from build123d import *

# Parameters (mm, degrees)
F0_R     = 20
F0_R_2   = 15
F1_DEPTH = 34
F2_R     = 22
F2_R_2   = 12
F3_DEPTH = 10.414


# Not quite as in the source:
# - a pattern or mirror of a feature is missing from the dataset's text; its kind, count and spacing are read off the source's solid


with BuildPart() as f1:
    # F0 (on Right) → F1 (new body, symmetric)
    with BuildSketch(Plane.YZ):
        Circle(F0_R)
        Circle(F0_R_2, mode=Mode.SUBTRACT)
    extrude(amount=F1_DEPTH, both=True)

    # F2 (on face) → F3 (join)
    with BuildSketch(Plane.YZ.offset(34)):
        Circle(F2_R)
        Circle(F2_R_2, mode=Mode.SUBTRACT)
    f3 = extrude(amount=F3_DEPTH)

    # F3_copies: F3 across plane
    add(f3.mirror(Plane(origin=(0, 0, 0), x_dir=(0, 0, -1), z_dir=(-1, 0, 0))))


solid = f1.part
Design review of the part built by this model. Coordinates are the model's own, in mm. A direction names the side the tool comes from. Give positions to 0.01 mm unless a question says otherwise; leave off trailing zeros. Write each loop counter-clockwise with the first axis right and the second up, starting at its lowest first coordinate (ties: lowest second). Pieces come first, ordered by that corner, then holes. Notation, with made-up numbers: M 53.25,64 L 111.25,64 A12 cw 111.25,70 Z; hole C -7.5,-5 d11. An arc over 180 degrees is marked long. Return JSON: item names as keys, results as strings. Group by question number.
Item 1: Clearance check with flat-ended pins moving along their axes: pin 1 Ø5 at (x, z) = (-33, -10.5) entering from +Y; pin 2 Ø6 at (x, z) = (30, -16.5) entering from -Y; pin 3 Ø4 at (x, y) = (9.5, -11) entering from -Z. State where each tip first meets the part, or that it passes through.
Item 2: Wall thickness on line 1 along Z through (x, y) = (-39, 0); line 2 along X through (y, z) = (-12.5, -2); line 3 along Z through (x, y) = (12, 0): over which ranges is each line inside the solid? List them lowest first.
Item 3: Take a section at A-A (z = 0). Give the boundary of the cut face in (x, y).
Item 4: Take a section at C-C (x = 7). Give the boundary of the cut face in (y, z).
Item 5: Take a section at D-D (y = -16). Give the boundary of the cut face in (x, z).
Item 6: Tool access review of faces 4 (the cylindrical face through (-39.13, -11.99, 0.53)), 5 (the flat face through (34, 10, -18)): name each direction out of +Z, -Z, +X, -X, +Y, -Y from which nothing blocks a thin tool from reaching the whole face with its end or side.
Item 7: The part is to be moulded in two halves that separate along Z. For faces 1 (the flat face through (34, -7, 10)), 2 (the cylindrical face through (39.134, -4.769, -21.477)), 3 (the flat face through (44.414, 9, -9)), say which applies: pulls with the +Z half, pulls with the -Z half, needs draft (parallel to the pull), parting line crosses it, or undercut.
Return value:
{
 "1": {"pin 1": "stops at y = 20.41", "pin 2": "stops at y = -14.76", "pin 3": "stops at z = -17.86"},
 "2": {"line 1": "z = -22 to -12, 12 to 22", "line 2": "x = -44.41 to -34, 34 to 44.41", "line 3": "z = -20 to -15, 15 to 20"},
 "3": {"outline": "M -44.41,-22 L -34,-22 L -34,-20 L 34,-20 L 34,-22 L 44.41,-22 L 44.41,-12 L 34,-12 L 34,-15 L -34,-15 L -34,-12 L -44.41,-12 Z; M -44.41,12 L -34,12 L -34,15 L 34,15 L 34,12 L 44.41,12 L 44.41,22 L 34,22 L 34,20 L -34,20 L -34,22 L -44.41,22 Z"},
 "4": {"outline": "C 0,0 d40; hole C 0,0 d30"},
 "5": {"outline": "M -44.41,-15.1 L -34,-15.1 L -34,-12 L 34,-12 L 34,-15.1 L 44.41,-15.1 L 44.41,15.1 L 34,15.1 L 34,12 L -34,12 L -34,15.1 L -44.41,15.1 Z"},
 "6": {"face 4": "+X, -X", "face 5": "none"},
 "7": {"face 1": "undercut", "face 2": "parting line crosses it", "face 3": "needs draft"}
}
